For this review, take the finished solid that the model builds, in its own axes (mm). Face numbers are marked on the shaded views. A direction names the side the tool comes from. Round coordinates to 2 decimals unless told otherwise and drop trailing zeros. Write each loop counter-clockwise with the first axis right and the second up, starting at its lowest first coordinate (ties: lowest second). Pieces come first, ordered by that corner, then holes.
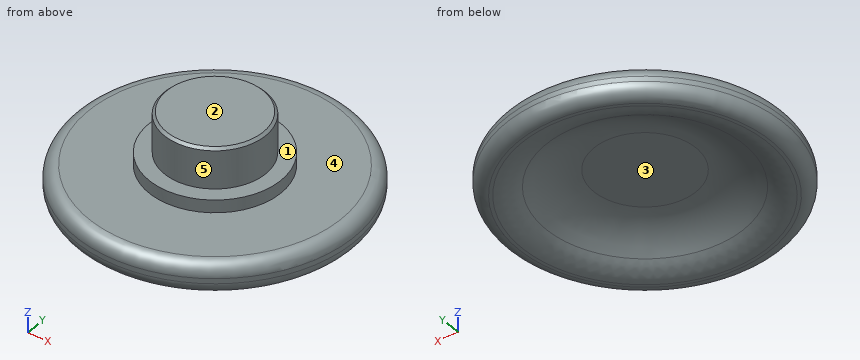
from build123d import *

# Parameters (mm, degrees)
F0_R     = 10.95
F1_DEPTH = 2.4
F2_R     = 4
F3_DEPTH = 4.2
F4_R     = 1
F5_R     = 5.2
F5_R_2   = 4
F6_DEPTH = 1
F7_R     = 1
F8_R     = 8.5
F9_DEPTH = 2
F11_SIZE = 0.2
F12_R    = 3


# Not quite as in the source:
# - a fillet or chamfer that OpenCascade refuses, or shapes differently, is made with other operations: its cross-section is extruded or revolved along the edge and cut away or added


with BuildPart() as f1:
    # F0 (on Top) → F1 (new body)
    with BuildSketch(Plane.XY):
        Circle(F0_R)
    extrude(amount=F1_DEPTH)

    # F2 (on face) → F3 (join)
    with BuildSketch(Plane.XY.offset(2.4)):
        Circle(F2_R)
    extrude(amount=F3_DEPTH)

    # F4
    f4_edges = [f1.edges().sort_by_distance(p)[0] for p in [
        (-10.95, 0, 2.4),
    ]]
    fillet(f4_edges, radius=F4_R)

    # F5 (on face) → F6 (join)
    with BuildSketch(Plane.XY.offset(2.4)):
        Circle(F5_R)
        Circle(F5_R_2, mode=Mode.SUBTRACT)
    extrude(amount=F6_DEPTH)

    # F7
    f7_edges = [f1.edges().sort_by_distance(p)[0] for p in [
        (-10.95, 0, 0),
    ]]
    fillet(f7_edges, radius=F7_R)

    # F8 (on face) → F9 (cut)
    with BuildSketch(Plane(origin=(0, 0, 0), x_dir=(1, 0, 0), z_dir=(0, 0, -1))):
        Circle(F8_R)
    extrude(amount=-F9_DEPTH, mode=Mode.SUBTRACT)

    # F10: fillet of radius 6 on 1 edges, made by hand

    # F10_s1 → F10_t2 (revolve)
    with BuildSketch(Plane.XZ):
        with BuildLine():
            ThreePointArc((8.5, 0), (6.4773537878, 1.4772255751), (4.027864045, 2))
            Line((4.027864045, 2), (8.5, 2))
            Line((8.5, 2), (8.5, 0))
        make_face()
    revolve(axis=Axis((0, 0, 2), (0, 0, -1)))

    # F11
    f11_edges = [f1.edges().sort_by_distance(p)[0] for p in [
        (-4, 0, 6.6),
    ]]
    chamfer(f11_edges, length=F11_SIZE)

    # F12
    f12_edges = [f1.edges().sort_by_distance(p)[0] for p in [
        (-8.5, 0, 0),
    ]]
    fillet(f12_edges, radius=F12_R)


solid = f1.part
(1) For the marked faces 1 and 2, list the 3-axis set-ups (+Z, -Z, +X, -X, +Y, -Y) from which the entire face can be reached by the end or side of a thin tool; tool diameter is ignored.
Geometry check:
face 1: +Z
face 2: +Z, +X, -X, +Y, -Y
(2) For line 1 along Z through (x, y) = (-3, -0.25); line 2 along X through (y, z) = (3, 0.5); line 3 along Y through (x, z) = (-1.25, 5), list the stretches that pass through material, from the lowest coordinate up.
Geometry check:
line 1: z = 2 to 6.6
line 2: x = -10.39 to -7.44, 7.44 to 10.39
line 3: y = -3.8 to 3.8
(3) For pin 1 Ø6.5 at (x, y) = (0.5, 2) entering from -Z; pin 2 Ø3 at (x, y) = (7, 7.5) entering from +Z, all flat-tipped, find the tip position at first contact; note any pin that passes through.
Geometry check:
pin 1: stops at z = 1.86
pin 2: stops at z = 2.4
(4) Mouldability with a two-part tool opening along Y and no side actions: class the marked faces 3, 4 and 5 as pulls with the +Y half, pulls with the -Y half, needs draft (parallel to the pull), parting line crosses it, or undercut.
Geometry check:
face 3: undercut
face 4: needs draft
face 5: parting line crosses it
(5) We need section A-A, the plane z = 3. Give the boundary of the cut face in (x, y), and give its area (3 significant figures).
Geometry check:
outline: circle Ø10.4 at (0, 0)
area: 84.9 mm2
